Geometry check sheet. Reference: drawing and pictorial views, mm from the part's lowest x, y, z. Round coordinates to 2 decimals unless told otherwise and drop trailing zeros. Write each loop counter-clockwise with the first axis right and the second up, starting at its lowest first coordinate (ties: lowest second). Pieces come first, ordered by that corner, then holes. Notation, with made-up numbers: M 23.25,1.5 L 45.25,1.5 A27 ccw 45.25,23.5 Z; hole C 23,15.5 d5. An arc over 180 degrees is marked long. Use a Markdown table: item, result. Add a question column.
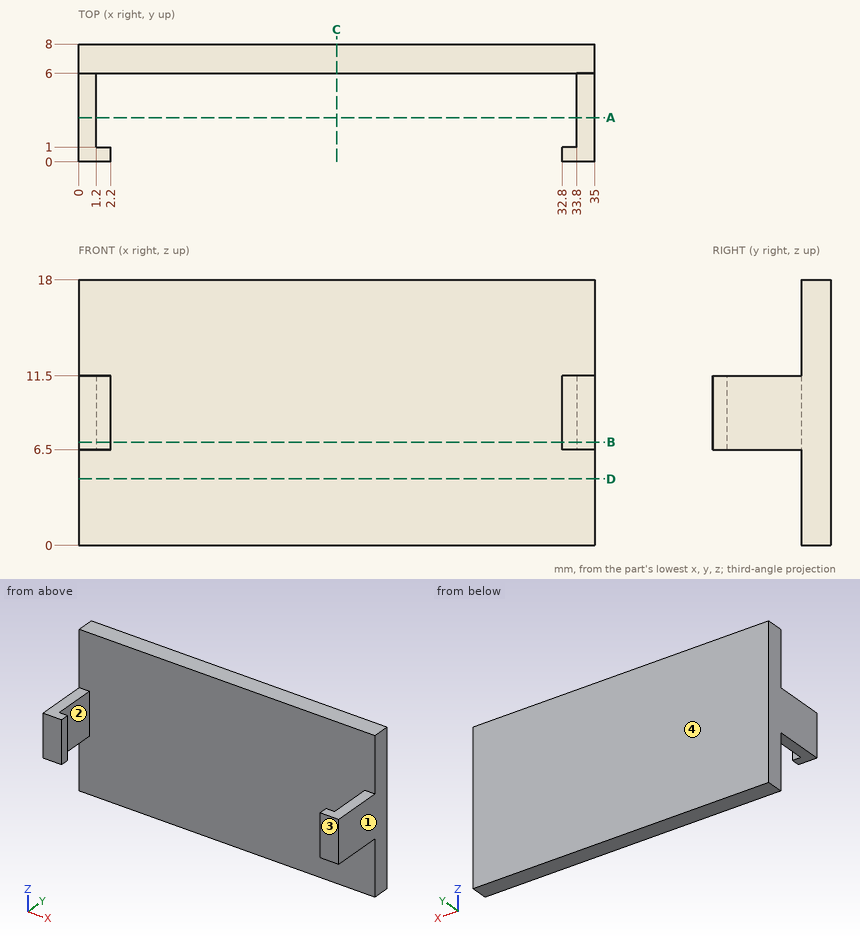
1. Cross-section at C-C on x = 17.5. Enter the section's corners in (y, z).
2. Cross-section at B-B on z = 7. Enter the section's corners in (x, y), plus the area to 3 significant figures.
3. Scan line: line 1 along Y through (x, z) = (15, 3.25). Record every from-to range of solid material in increasing order. Write a range as from..to.
4. Cross-section at A-A on y = 3. Enter the section's corners in (x, z), plus the area to 3 significant figures.
5. Depth check by flat-ended pin: pin 1 Ø2.5 at (x, y) = (0.5, 4) entering from -Z; pin 2 Ø1 at (x, y) = (10.5, 5) entering from -Z; pin 3 Ø1.1 at (x, y) = (1.5, 2.5) entering from +Z; pin 4 Ø5.5 at (x, z) = (21, 5.5) entering from -Y. Enter the tip coordinate at first touch or a pass-through.
6. Release check for a two-part mould opening along Y. For the marked faces 1, 2, 3 and 4 record: +Y half, -Y half, draft (parallel to the pull), parting line (faces both ways), or undercut.
7. Cross-section at D-D on z = 4.5. Enter the section's corners in (x, y), plus the area to 3 significant figures.
Answer:
| question | item | result |
|---|---|---|
| 1 | outline | M 6,0 L 8,0 L 8,18 L 6,18 Z |
| 2 | outline | M 0,0 L 2.2,0 L 2.2,1 L 1.2,1 L 1.2,6 L 33.8,6 L 33.8,1 L 32.8,1 L 32.8,0 L 35,0 L 35,8 L 0,8 Z |
| 2 | area | 86.4 mm^2 |
| 3 | line 1 | y = 6..8 |
| 4 | outline | M 0,6.5 L 1.2,6.5 L 1.2,11.5 L 0,11.5 Z; M 33.8,6.5 L 35,6.5 L 35,11.5 L 33.8,11.5 Z |
| 4 | area | 12.0 mm^2 |
| 5 | pin 1 | stops at z = 6.5 |
| 5 | pin 2 | passes through |
| 5 | pin 3 | stops at z = 11.5 |
| 5 | pin 4 | stops at y = 6 |
| 6 | face 1 | draft |
| 6 | face 2 | undercut |
| 6 | face 3 | -Y half |
| 6 | face 4 | +Y half |
| 7 | outline | M 0,6 L 35,6 L 35,8 L 0,8 Z |
| 7 | area | 70.0 mm^2 |
